Verification items for the finished model (mm, model axes). A direction names the side the tool comes from. Give positions to 0.01 mm unless a question says otherwise; leave off trailing zeros. Loops run counter-clockwise (first coordinate to the right, second up) from the corner with the lowest first, then second, coordinate; pieces in that order, holes last. Notation, with made-up numbers: M 87,-34.5 L 133,-34.5 A16 cw 133,-27.5 Z; hole C -0.75,84.5 d2. An arc over 180 degrees is marked long. Use a Markdown table: item, result.
Solid Edge part; units mm, degrees
sketch "Sketch1" plane through (0, 0, 0) normal (0, -1, 0) x (1, 0, 0)
  line L0 (47.5, 4) -> (47.5, 0)
  line L1 (47.5, 0) -> (75, 0)
  line L2 (75, 0) -> (75, 8)
  line L3 (75, 8) -> (52.5, 8)
  line L4 (52.5, 8) -> (52.5, 8.5)
  line L5 (52.5, 8.5) -> (50, 8.5)
  line L6 (50, 8.5) -> (50, 4)
  line L7 (50, 4) -> (47.5, 4)
  dimension "D1" = 47.5
  dimension "D2" = 75
revolve "RevolvedProtrusion1" add sketch "Sketch1" angle 360 about axis through (0, 0, 54) along (0, 0, -1)
hole "Hole_1" at (64.2607, 0, 0) direction (0, 0, 1) diameter 4.8 end up to next counterbore diameter 8 counterbore depth 4.8
pattern_circular "Pattern1" count 5 over 360 about axis through (0, 0, 8) along (0, 0, 1) of "Hole_1"
hole "Hole_2" at (-65, 0, 0) direction (0, 0, 1) diameter 7 end up to next
pattern_circular "Pattern2" count 5 over 360 about axis through (0, 0, 0) along (0, 0, 1) of "Hole_2"
properties material "Polyethylene, low density"
(1) Cross-section at D-D on y = 29. Record the cut outline in (x, z).
Results below:
| item | result |
|---|---|
| outline | M -69.17,0 L -37.62,0 L -37.62,4 L -40.73,4 L -40.73,8.5 L -43.76,8.5 L -43.76,8 L -69.17,8 Z; M 37.62,0 L 69.17,0 L 69.17,8 L 43.76,8 L 43.76,8.5 L 40.73,8.5 L 40.73,4 L 37.62,4 Z |
(2) Gauge pin test, flat ends, axial feed: P1, Ø2, axis at x = 41, z = 1, coming from the -Y side; P2, Ø2.5, axis at x = 20.5, y = 59.5, coming from the -Z side; P3, Ø1.5, axis at y = 43, z = 7.5, coming from the +X side; P4, Ø5.5, axis at x = 52.59, y = -38.21, coming from the -Z side. Record the tip position at first contact, or that the pin passes through.
Results below:
| item | result |
|---|---|
| P1 | y = -63.44 |
| P2 | z = 4.8 |
| P3 | x = 61.97 |
| P4 | through |
(3) Set-up check for faces 1 (the cylindrical face through (-52.55, 35.44, 6.38)), 2 (the flat face through (44.2, 18.3, 4)), 3 (the flat face through (-53.5, 35.6, 4.8)): record each of +Z, -Z, +X, -X, +Y, -Y from which the full face is reachable in a straight line by a thin tool's end or side.
Results below:
| item | result |
|---|---|
| face 1 | +Z, -Z |
| face 2 | +Z |
| face 3 | -Z |
(4) Draft check along X on faces 4 (the flat face through (46.4, 19.2, 8.5)), 5 (the cylindrical face through (50.076, 15.77, 8.254)), 6 (the flat face through (17, 62, 4.8)), 7 (the cylindrical face through (19.26, 63.44, 6.38)). Enter one of: +X half, -X half, draft (parallel to the pull), parting line (faces both ways), or undercut.
Results below:
| item | result |
|---|---|
| face 4 | draft |
| face 5 | parting line |
| face 6 | undercut |
| face 7 | undercut |
(5) Material ranges on line 1 (X direction, y = 0, z = 1.8); line 2 (X direction, y = 0, z = 7.25); line 3 (Y direction, x = 49.5, z = 0.5) (3 decimals), recorded low to high.
Results below:
| item | result |
|---|---|
| line 1 | -75 to -68.5, -61.5 to -47.5, 47.5 to 60.26, 68.26 to 75 |
| line 2 | -75 to -68.5, -61.5 to -50, 50 to 61.86, 66.66 to 75 |
| line 3 | -56.345 to -39.857, -36.555 to 36.555, 39.857 to 56.345 |
(6) Cross-section at A-A on y = 0. Record the cut outline in (x, z), then the cut area to 3 significant figures.
Results below:
| item | result |
|---|---|
| outline | M -75,0 L -68.5,0 L -68.5,8 L -75,8 Z; M -61.5,0 L -47.5,0 L -47.5,4 L -50,4 L -50,8.5 L -52.5,8.5 L -52.5,8 L -61.5,8 Z; M 47.5,0 L 60.26,0 L 60.26,4.8 L 61.86,4.8 L 61.86,8 L 52.5,8 L 52.5,8.5 L 50,8.5 L 50,4 L 47.5,4 Z; M 66.66,4.8 L 68.26,4.8 L 68.26,0 L 75,0 L 75,8 L 66.66,8 Z |
| area | 313 mm^2 |
(7) Cross-section at C-C on z = 2. State how many separate pieces and enclosed holes the cut face has, then the cut area to 3 significant figures.
Results below:
| item | result |
|---|---|
| separate pieces | 1 |
| enclosed holes | 11 |
| area | 10,100 mm^2 |
(8) Cross-section at B-B on x = -65. Record the cut outline in (y, z), then the cut area to 3 significant figures.
Results below:
| item | result |
|---|---|
| outline | M -37.42,0 L -3.5,0 L -3.5,8 L -37.42,8 Z; M 3.5,0 L 37.42,0 L 37.42,8 L 3.5,8 Z |
| area | 543 mm^2 |
